Could you check a few things on this model? Use its own coordinates, in mm. A direction names the side the tool comes from. Round coordinates to 2 decimals unless told otherwise and drop trailing zeros. Write each loop counter-clockwise with the first axis right and the second up, starting at its lowest first coordinate (ties: lowest second). Pieces come first, ordered by that corner, then holes. Notation, with made-up numbers: M -6,14.5 L -1,14.5 A18 ccw -1,28.5 Z; hole C 66,49.5 d10. An arc over 180 degrees is marked long. One line per question, with ' | ' between items. Start each with the question number.
```python
from build123d import *

# Parameters (mm, degrees)
BASPROSKE_W         = 15
BASPROSKE_H         = 13.42
TOOTHCUT_DEPTH      = 25.190758566
TEETHCUTS_COUNT     = 20
TEETHCUTS_ANGLE     = 342
BORSKE_R            = 4
BORE_DEPTH          = 50.0000508
BOSS_EXTRUDE1_START = -15
BOSS_EXTRUDE1_DEPTH = 15
SKETCH2_W           = 1.2
SKETCH2_H           = 8
CUT_EXTRUDE1_DEPTH  = 2


with BuildPart() as part:
    # BasProSke → Base-Revolve (revolve)
    with BuildSketch(Plane(origin=(0, 0, 0), x_dir=(1, 0, 0), z_dir=(0, 1, 0)), mode=Mode.PRIVATE) as base_revolve_sk:
        with Locations((7.5, 6.71)):
            Rectangle(BASPROSKE_W, BASPROSKE_H)
    revolve(base_revolve_sk.sketch.rotate(Axis((-10, 0, 0), (1, 0, 0)), 180), axis=Axis((-10, 0, 0), (1, 0, 0)))

    # TooCutSke → ToothCut (cut, through all)
    with BuildSketch(Plane(origin=(0, 0, 0), x_dir=(0, 0, -1), z_dir=(1, 0, 0))):
        with BuildLine():
            ThreePointArc((0.607848894, 10.656678456), (0, 10.674), (-0.607848894, 10.656678456))
            ThreePointArc((-0.607848894, 10.656678456), (-1.001950595, 12.081933102), (-1.804853959, 13.32371132))
            ThreePointArc((-1.804853959, 13.32371132), (0, 13.4454), (1.804853959, 13.32371132))
            ThreePointArc((1.804853959, 13.32371132), (1.001950595, 12.081933102), (0.607848894, 10.656678456))
        make_face()
    toothcut = extrude(amount=TOOTHCUT_DEPTH, mode=Mode.SUBTRACT)

    # TeethCuts: ToothCut ×20 about axis
    teethcuts_axis = Axis((-10, 0, 0), (1, 0, 0))
    for i in range(1, TEETHCUTS_COUNT):
        add(toothcut.rotate(teethcuts_axis, i * TEETHCUTS_ANGLE / (TEETHCUTS_COUNT - 1)), mode=Mode.SUBTRACT)

    # BorSke → Bore (cut, symmetric)
    with BuildSketch(Plane(origin=(0, 0, 0), x_dir=(0, 0, -1), z_dir=(1, 0, 0))):
        with Locations(Location((0, 0, 0), (0, 0, 180))):
            Circle(BORSKE_R)
    extrude(amount=BORE_DEPTH, both=True, mode=Mode.SUBTRACT)

    # Sketch1 → Boss-Extrude1 (add)
    with BuildSketch(Plane.ZY.offset(BOSS_EXTRUDE1_START)):
        with BuildLine():
            Line((-2.856571371, 2.8), (2.856571371, 2.8))
            ThreePointArc((2.856571371, 2.8), (0, 4), (-2.856571371, 2.8))
        make_face()
    extrude(amount=BOSS_EXTRUDE1_DEPTH)

    # Sketch2 → Cut-Extrude1 (cut)
    with BuildSketch(Plane.ZY):
        with Locations((-7, 0)):
            Rectangle(SKETCH2_W, SKETCH2_H)
    extrude(amount=-CUT_EXTRUDE1_DEPTH, mode=Mode.SUBTRACT)


solid = part.part
```
1. Suppose I cut it at A-A (y = 0). Write out the boundary of the cut face in (x, z), and give its area (3 significant figures).
2. I'm going to push flat-ended pins straight in: P1, Ø0.6, axis at y = -1, z = -7, coming from the -X side; P2, Ø8, axis at x = 9, y = -5.5, coming from the -Z side; P3, Ø1, axis at x = 0.5, y = -1, coming from the -Z side. Where does each tip first touch, or does it pass through?
3. Which directions (+Z, -Z, +X, -X, +Y, -Y) give clear straight access to the entire face, cutting with the end or side of a thin tool? Please do faces 1 (the face through (2, 0, -7)), 2 (the face through (7.395, -12.049, -0.987)), 3 (the face through (7.395, -0.987, 12.049)), 4 (the face through (7.395, -2.784, -11.765)).
4. Suppose I cut it at C-C (z = -7.25). Write out the boundary of the cut face in (x, y).
5. If we mould it in two halves opening along Y, with no side actions, what happens to faces 5 (the face through (7.395, -10.328, 6.284)), 6 (the face through (7.395, 12.049, 0.987)), 7 (the face through (7.395, -9.168, -7.881))? For each: released by +Y, released by -Y, zero draft, split by the parting line, or undercut.
6. I need wall thicknesses on line 1 along Z through (x, y) = (5, 0); line 2 along Y through (x, z) = (11, 0); line 3 along Y through (x, z) = (13.5, -8.75). Which ranges of each line are inside material? Lowest first, please. Write a range as from..to.
7. Suppose I cut it at B-B (z = 0). Write out the boundary of the cut face in (x, y).
8. Suppose I cut it at D-D (z = -3.25). Write out the boundary of the cut face in (x, y), and give its area (3 significant figures).
Computed:
1) outline: M 0,-10.67 L 15,-10.67 L 15,-4 L 0,-4 L 0,-6.4 L 2,-6.4 L 2,-7.6 L 0,-7.6 Z; M 0,4 L 15,4 L 15,10.67 L 0,10.67 Z | area: 198 mm²
2) P1: stops at x = 2 | P2: stops at z = -13.3 | P3: stops at z = -12.94
3) face 1: -X | face 2: +X, -X, -Y | face 3: +Z, +X, -X | face 4: +X, -X
4) outline: M 0,-8.73 L 15,-8.73 L 15,8.73 L 0,8.73 L 0,4 L 2,4 L 2,-4 L 0,-4 Z
5) face 5: undercut | face 6: released by +Y | face 7: released by -Y
6) line 1: z = -10.67..-4, 4..10.67 | line 2: y = -10.67..-4, 2.8..10.67 | line 3: y = -9.57..-7.28, -6.11..6.11, 7.28..9.57
7) outline: M 0,-10.67 L 15,-10.67 L 15,-4 L 0,-4 Z; M 0,2.8 L 15,2.8 L 15,10.67 L 0,10.67 Z
8) outline: M 0,-10.17 L 15,-10.17 L 15,-2.33 L 0,-2.33 Z; M 0,2.33 L 15,2.33 L 15,10.17 L 0,10.17 Z | area: 235 mm²
